Geometry: final body of the model. Coordinates: model frame, mm. Face numbers are marked on the shaded views. A direction names the side the tool comes from. Give positions to 0.01 mm unless a question says otherwise; leave off trailing zeros. Write each loop counter-clockwise with the first axis right and the second up, starting at its lowest first coordinate (ties: lowest second). Pieces come first, ordered by that corner, then holes. Notation, with made-up numbers: (28.25, 81.25) -> (60.25, 81.25) arc R23 ccw to (60.25, 107.25) -> close; hole circle Ø2 at (-24, 28.25). An arc over 180 degrees is marked (long way). Answer in a Markdown table with one row per item. Add a question column.
Item 1: Access query for the marked faces 5, 6, 7 and 8. Directions: +Z, -Z, +X, -X, +Y, -Y. A direction counts if a zero-diameter tool reaches every point of the face in a straight line with its end or side. Return the directions, or none.
Item 2: Section query A-A on y = 7. Output: boundary loops of the cut face in (x, z), plus the area to 3 significant figures.
Item 3: Section query B-B on x = -23. Output: boundary loops of the cut face in (y, z).
Item 4: First-contact query: P1, Ø2.5, axis at y = -12.5, z = 2.5, coming from the -X side; P2, Ø1, axis at y = 4, z = 3, coming from the +X side; P3, Ø1.2, axis at x = 23, z = 2, coming from the +Y side; P4, Ø12, axis at x = -4, y = -3.5, coming from the -Z side. Flat tips, straight axial feed; report the tip coordinate or a pass-through.
Item 5: Section query C-C on y = 27.5. Output: boundary loops of the cut face in (x, z), plus the area to 3 significant figures.
Item 6: Material intervals for probe 1 along X at (y, z) = (-2.5, 3.45); probe 2 along X at (y, z) = (12, 3.4); probe 3 along Y at (x, z) = (-12, 4.4), sorted ascending. Write a range as from..to.
Item 7: Draft query along X for the marked faces 1, 2, 3 and 4. Return one class per face: +X half, -X half, draft (parallel to the pull), parting line (faces both ways), or undercut.
```python
from build123d import *

# Parameters (mm, degrees)
SKETCH1_W           = 32
SKETCH1_H           = 34.840049923
BOSS_EXTRUDE1_DEPTH = 5


with BuildPart() as part:
    # Sketch1 → Boss-Extrude1 (new body)
    with BuildSketch(Plane.XY):
        with BuildLine():
            Line((-27, 10), (-27, 15))
            Line((-27, 15), (-33.823069051, 15))
            ThreePointArc((-33.823069051, 15), (0, 37), (33.823069051, 15))
            Line((33.823069051, 15), (27, 15))
            Line((27, 15), (27, 10))
            Line((27, 10), (32, 10))
            Line((32, 10), (32, 5))
            Line((32, 5), (27, 5))
            Line((27, 5), (27, 1.5))
            Line((27, 1.5), (24, 1.5))
            Line((24, 1.5), (24, 2.6))
            Line((24, 2.6), (21.7, 2.6))
            Line((21.7, 2.6), (21.7, 1.5))
            Line((21.7, 1.5), (17, 1.5))
            Line((17, 1.5), (17, -1.5))
            Line((17, -1.5), (21.7, -1.5))
            Line((21.7, -1.5), (21.7, -2.6))
            Line((21.7, -2.6), (24, -2.6))
            Line((24, -2.6), (24, -1.5))
            Line((24, -1.5), (27, -1.5))
            Line((27, -1.5), (27, -5))
            Line((27, -5), (32, -5))
            Line((32, -5), (32, -10))
            Line((32, -10), (27, -10))
            Line((27, -10), (27, -15))
            Line((27, -15), (33.823069051, -15))
            ThreePointArc((33.823069051, -15), (26.162950904, -26.162950904), (15, -33.823069051))
            Line((15, -33.823069051), (15, -27))
            Line((15, -27), (10, -27))
            Line((10, -27), (10, -32))
            Line((10, -32), (5, -32))
            Line((5, -32), (5, -27))
            Line((5, -27), (1.5, -27))
            Line((1.5, -27), (1.5, -24))
            Line((1.5, -24), (2.6, -24))
            Line((2.6, -24), (2.6, -21.7))
            Line((2.6, -21.7), (1.5, -21.7))
            Line((1.5, -21.7), (1.5, -17))
            Line((1.5, -17), (-1.5, -17))
            Line((-1.5, -17), (-1.5, -21.7))
            Line((-1.5, -21.7), (-2.6, -21.7))
            Line((-2.6, -21.7), (-2.6, -24))
            Line((-2.6, -24), (-1.5, -24))
            Line((-1.5, -24), (-1.5, -27))
            Line((-1.5, -27), (-5, -27))
            Line((-5, -27), (-5, -32))
            Line((-5, -32), (-10, -32))
            Line((-10, -32), (-10, -27))
            Line((-10, -27), (-15, -27))
            Line((-15, -27), (-15, -33.823069051))
            ThreePointArc((-15, -33.823069051), (-26.162950904, -26.162950904), (-33.823069051, -15))
            Line((-33.823069051, -15), (-27, -15))
            Line((-27, -15), (-27, -10))
            Line((-27, -10), (-32, -10))
            Line((-32, -10), (-32, -5))
            Line((-32, -5), (-27, -5))
            Line((-27, -5), (-27, -1.5))
            Line((-27, -1.5), (-24, -1.5))
            Line((-24, -1.5), (-24, -2.6))
            Line((-24, -2.6), (-21.7, -2.6))
            Line((-21.7, -2.6), (-21.7, -1.5))
            Line((-21.7, -1.5), (-17, -1.5))
            Line((-17, -1.5), (-17, 1.5))
            Line((-17, 1.5), (-21.7, 1.5))
            Line((-21.7, 1.5), (-21.7, 2.6))
            Line((-21.7, 2.6), (-24, 2.6))
            Line((-24, 2.6), (-24, 1.5))
            Line((-24, 1.5), (-27, 1.5))
            Line((-27, 1.5), (-27, 5))
            Line((-27, 5), (-32, 5))
            Line((-32, 5), (-32, 10))
            Line((-32, 10), (-27, 10))
        make_face()
        with Locations((0, 7.420024962)):
            Rectangle(SKETCH1_W, SKETCH1_H, mode=Mode.SUBTRACT)
    extrude(amount=BOSS_EXTRUDE1_DEPTH)


solid = part.part
```
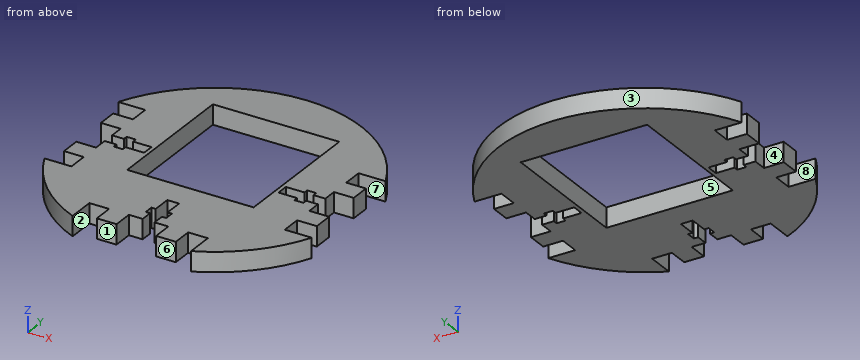
Findings below:
| question | item | result |
|---|---|---|
| 1 | face 5 | +Z, -Z |
| 1 | face 6 | +Z, -Z, -Y |
| 1 | face 7 | +Z, -Z, +X |
| 1 | face 8 | +Z, -Z, -X |
| 2 | outline | (-32, 0) -> (-16, 0) -> (-16, 5) -> (-32, 5) -> close; (16, 0) -> (32, 0) -> (32, 5) -> (16, 5) -> close |
| 2 | area | 160 mm^2 |
| 3 | outline | (-28.98, 0) -> (-2.6, 0) -> (-2.6, 5) -> (-28.98, 5) -> close; (2.6, 0) -> (28.98, 0) -> (28.98, 5) -> (2.6, 5) -> close |
| 4 | P1 | stops at x = -27 |
| 4 | P2 | stops at x = 27 |
| 4 | P3 | stops at y = 29.45 |
| 4 | P4 | passes through |
| 5 | outline | (-24.75, 0) -> (24.75, 0) -> (24.75, 5) -> (-24.75, 5) -> close |
| 5 | area | 248 mm^2 |
| 6 | probe 1 | x = -27..-24, -21.7..-16, 16..21.7, 24..27 |
| 6 | probe 2 | x = -27..-16, 16..27 |
| 6 | probe 3 | y = -27..-10, 24.84..35 |
| 7 | face 1 | undercut |
| 7 | face 2 | undercut |
| 7 | face 3 | parting line |
| 7 | face 4 | draft |
